Design review of the part built by this model. Coordinates are the model's own, in mm. A direction names the side the tool comes from. Coordinates: 2 decimals unless noted, no trailing zeros. Write each loop counter-clockwise with the first axis right and the second up, starting at its lowest first coordinate (ties: lowest second). Pieces come first, ordered by that corner, then holes. Notation, with made-up numbers: M 83,46.5 L 93,46.5 A28 cw 93,65.5 Z; hole C -20.75,22 d3. An arc over 180 degrees is marked long. One line per question, with ' | ' between items.
from build123d import *

# Parameters (mm, degrees)
ESBO_O1_W                = 44
ESBO_O1_H                = 30
ESBO_O1_W_2              = 40
ESBO_O1_H_2              = 26
RESSALTO_EXTRUS_O1_DEPTH = 20
ESBO_O3_W                = 15
ESBO_O3_H                = 26
CORTE_EXTRUS_O1_DEPTH    = 20
ESBO_O4_W                = 44
ESBO_O4_H                = 30
RESSALTO_EXTRUS_O2_DEPTH = 2
ESBO_O5_R                = 1.6
CORTE_EXTRUS_O2_DEPTH    = 2


with BuildPart() as part:
    # Esboço1 → Ressalto-extrusão1 (new body)
    with BuildSketch(Plane.XY):
        with Locations((22, 15)):
            Rectangle(ESBO_O1_W, ESBO_O1_H)
        with Locations((22, 15)):
            Rectangle(ESBO_O1_W_2, ESBO_O1_H_2, mode=Mode.SUBTRACT)
    extrude(amount=RESSALTO_EXTRUS_O1_DEPTH)

    # Esboço3 → Corte-extrusão1 (cut)
    with BuildSketch(Plane.ZY):
        with Locations((7.5, 15)):
            Rectangle(ESBO_O3_W, ESBO_O3_H)
    extrude(amount=-CORTE_EXTRUS_O1_DEPTH, mode=Mode.SUBTRACT)

    # Esboço4 → Ressalto-extrusão2 (add)
    with BuildSketch(Plane.XY.offset(20)):
        with Locations((22, 15)):
            Rectangle(ESBO_O4_W, ESBO_O4_H)
    extrude(amount=-RESSALTO_EXTRUS_O2_DEPTH)

    # Esboço5 → Corte-extrusão2 (cut)
    with BuildSketch(Plane.XY.offset(20)):
        with Locations((38.47, 25.04)):
            Circle(ESBO_O5_R)
        with Locations(Location((38.47, 4.96, 0), (0, 0, 180))):
            Circle(ESBO_O5_R)
    extrude(amount=-CORTE_EXTRUS_O2_DEPTH, mode=Mode.SUBTRACT)


solid = part.part
1. Take a section at D-D (z = 6.5). Write out the cut boundary in (x, y), then the cut area to 3 significant figures.
Answer sheet:
outline: M 0,0 L 44,0 L 44,30 L 0,30 L 0,28 L 42,28 L 42,2 L 0,2 Z | area: 228 mm^2
2. Take a section at C-C (x = 38.47). Write out the cut boundary in (y, z).
Answer sheet:
outline: M 0,0 L 2,0 L 2,18 L 3.36,18 L 3.36,20 L 0,20 Z; M 6.56,18 L 23.44,18 L 23.44,20 L 6.56,20 Z; M 26.64,18 L 28,18 L 28,0 L 30,0 L 30,20 L 26.64,20 Z
3. Draft analysis for pull direction Y (two halves, no side actions). For faces 1 (the face through (2, 15, 16)), 2 (the face through (22, 30, 10)), 3 (the face through (21, 2, 9)), 4 (the face through (44, 15, 10)), state which applies: pulls with the +Y half, pulls with the -Y half, needs draft (parallel to the pull), parting line crosses it, or undercut.
Answer sheet:
face 1: undercut | face 2: pulls with the +Y half | face 3: undercut | face 4: needs draft
4. To check wall thickness, follow line 1 along Y through (x, z) = (38.47, 19.45); line 2 along Y through (x, z) = (16.5, 6.25); line 3 along X through (y, z) = (4.96, 19.6). State the ranges of each line that lie inside material, in increasing order. Write a range as [from, to].
Answer sheet:
line 1: [0, 3.36], [6.56, 23.44], [26.64, 30] | line 2: [0, 2], [28, 30] | line 3: [0, 36.87], [40.07, 44]
5. Tool access review of faces 5 (the face through (22, 15, 18)), 6 (the face through (36.944, 4.479, 19.014)), 7 (the face through (1, 15, 15)): name each direction out of +Z, -Z, +X, -X, +Y, -Y from which nothing blocks a thin tool from reaching the whole face with its end or side.
Answer sheet:
face 5: -Z | face 6: +Z, -Z | face 7: -Z, -X
6. Insertion check: pin 1 Ø1.5 at (x, y) = (36.5, 13) entering from -Z; pin 2 Ø5.5 at (y, z) = (19, 10) entering from -X; pin 3 Ø10 at (y, z) = (17.5, 17) entering from -X; pin 4 Ø1.6 at (x, y) = (1, 10.5) entering from -Z. Each pin has a flat end and moves straight along its axis. Give the tip position at first contact, or say it passes through.
Answer sheet:
pin 1: z = 18 | pin 2: x = 42 | pin 3: x = 0 | pin 4: z = 15
7. Take a section at B-B (y = 4.96). Write out the cut boundary in (x, z).
Answer sheet:
outline: M 0,15 L 2,15 L 2,18 L 36.87,18 L 36.87,20 L 0,20 Z; M 40.07,18 L 42,18 L 42,0 L 44,0 L 44,20 L 40.07,20 Z
8. Take a section at A-A (z = 16). Write out the cut boundary in (x, y).
Answer sheet:
outline: M 0,0 L 44,0 L 44,30 L 0,30 Z; hole M 2,2 L 42,2 L 42,28 L 2,28 Z
